```python
from build123d import *

# Parameters (mm, degrees)
BOSS_EXTRUDE1_DEPTH = 6.18
SKETCH2_R           = 2.1
CUT_EXTRUDE1_DEPTH  = 45.955560266
FILLET1_R           = 2
SKETCH3_R           = 1.16
BOSS_EXTRUDE2_DEPTH = 2
SKETCH5_W           = 46.23261583
SKETCH5_H           = 41.700006435
CUT_EXTRUDE2_DEPTH  = 6.18
SKETCH9_R           = 1.3
CUT_EXTRUDE3_DEPTH  = 39.857224753


with BuildPart() as part:
    # Sketch1 → Boss-Extrude1 (new body)
    with BuildSketch(Plane.XY):
        Polygon((0, 0), (0, 10), (7.5, 10), (12.499244943, 14.999244943), (12.499244943, 34.4), (24.749244943, 34.4), (24.749244943, 14.999244943), (29.748489886, 10), (37.248489886, 10), (37.248489886, 0), align=None)
    extrude(amount=BOSS_EXTRUDE1_DEPTH)

    # Sketch2 → Cut-Extrude1 (cut, through all)
    with BuildSketch(Plane(origin=(0, 10, 0), x_dir=(1, 0, 0), z_dir=(0, 1, 0))):
        with Locations(Location((3.75, -3.09, 0), (0, 0, 270))):
            Circle(SKETCH2_R)
        with Locations(Location((33.498489886, -3.09, 0), (0, 0, 270))):
            Circle(SKETCH2_R)
    extrude(amount=-CUT_EXTRUDE1_DEPTH, mode=Mode.SUBTRACT)

    # Fillet1
    fillet1_edges = [part.edges().sort_by_distance(p)[0] for p in [
        (0, 5, 0),
        (37.248489886, 5, 0),
        (12.499244943, 34.4, 3.09),
        (24.749244943, 34.4, 3.09),
        (0, 5, 6.18),
        (37.248489886, 5, 6.18),
    ]]
    fillet(fillet1_edges, radius=FILLET1_R)

    # Sketch3 → Boss-Extrude2 (add)
    # profile 1 of 15: a face of its own
    with BuildSketch(Plane(origin=(0, 0, 0), x_dir=(-1, 0, 0), z_dir=(0, 0, -1))):
        with BuildLine():
            Line((-14.76314253, 29.959470635), (-15.91314253, 29.959470635))
            ThreePointArc((-15.91314253, 29.959470635), (-18.51314253, 27.359470635), (-21.11314253, 29.959470635))
            Line((-21.11314253, 29.959470635), (-21.11314253, 21.454771123))
            Line((-21.11314253, 21.454771123), (-12.499244943, 21.454771123))
            Line((-12.499244943, 21.454771123), (-12.499244943, 22.849229594))
            ThreePointArc((-12.499244943, 22.849229594), (-13.32314253, 23.959470635), (-12.499244943, 25.069711675))
            Line((-12.499244943, 25.069711675), (-12.499244943, 27.381286163))
            ThreePointArc((-12.499244943, 27.381286163), (-14.116839829, 28.243933732), (-14.76314253, 29.959470635))
        make_face()
        with Locations((-18.51314253, 23.959470635)):
            Circle(SKETCH3_R, mode=Mode.SUBTRACT)
    # profile 2 of 15: a face of its own
    with BuildSketch(Plane(origin=(0, 0, 0), x_dir=(-1, 0, 0), z_dir=(0, 0, -1))):
        with BuildLine():
            ThreePointArc((-9.56314253, 29.959470635), (-10.447605628, 28.005773335), (-12.499244943, 27.381286163))
            Line((-12.499244943, 27.381286163), (-12.499244943, 25.069711675))
            ThreePointArc((-12.499244943, 25.069711675), (-11.47186791, 24.890995943), (-11.00314253, 23.959470635))
            ThreePointArc((-11.00314253, 23.959470635), (-11.47186791, 23.027945327), (-12.499244943, 22.849229594))
            Line((-12.499244943, 22.849229594), (-12.499244943, 21.454771123))
            Line((-12.499244943, 21.454771123), (-9.56314253, 21.454771123))
            Line((-9.56314253, 21.454771123), (-9.56314253, 29.959470635))
        make_face()
    # profile 3 of 15: a face of its own
    with BuildSketch(Plane(origin=(0, 0, 0), x_dir=(-1, 0, 0), z_dir=(0, 0, -1))):
        with BuildLine():
            Line((-13.31814253, 29.959470635), (-14.76314253, 29.959470635))
            ThreePointArc((-14.76314253, 29.959470635), (-14.116839829, 28.243933732), (-12.499244943, 27.381286163))
            Line((-12.499244943, 27.381286163), (-12.499244943, 28.854454722))
            ThreePointArc((-12.499244943, 28.854454722), (-13.091103544, 29.271783673), (-13.31814253, 29.959470635))
        make_face()
    # profile 4 of 15: a face of its own
    with BuildSketch(Plane(origin=(0, 0, 0), x_dir=(-1, 0, 0), z_dir=(0, 0, -1))):
        with BuildLine():
            Line((-12.499244943, 28.854454722), (-12.499244943, 27.381286163))
            ThreePointArc((-12.499244943, 27.381286163), (-10.447605628, 28.005773335), (-9.56314253, 29.959470635))
            Line((-9.56314253, 29.959470635), (-11.00814253, 29.959470635))
            ThreePointArc((-11.00814253, 29.959470635), (-11.475455569, 29.031509621), (-12.499244943, 28.854454722))
        make_face()
    # profile 5 of 15: a face of its own
    with BuildSketch(Plane(origin=(0, 0, 0), x_dir=(-1, 0, 0), z_dir=(0, 0, -1))):
        with BuildLine():
            Line((-13.31814253, 29.959470635), (-14.76314253, 29.959470635))
            ThreePointArc((-14.76314253, 29.959470635), (-14.116839829, 28.243933732), (-12.499244943, 27.381286163))
            Line((-12.499244943, 27.381286163), (-12.499244943, 28.854454722))
            ThreePointArc((-12.499244943, 28.854454722), (-13.091103544, 29.271783673), (-13.31814253, 29.959470635))
        make_face()
    # profile 6 of 15: a face of its own
    with BuildSketch(Plane(origin=(0, 0, 0), x_dir=(-1, 0, 0), z_dir=(0, 0, -1))):
        with BuildLine():
            Line((-12.499244943, 28.854454722), (-12.499244943, 27.381286163))
            ThreePointArc((-12.499244943, 27.381286163), (-10.447605628, 28.005773335), (-9.56314253, 29.959470635))
            Line((-9.56314253, 29.959470635), (-11.00814253, 29.959470635))
            ThreePointArc((-11.00814253, 29.959470635), (-11.475455569, 29.031509621), (-12.499244943, 28.854454722))
        make_face()
    # profile 7 of 15: a face of its own
    with BuildSketch(Plane(origin=(0, 0, 0), x_dir=(-1, 0, 0), z_dir=(0, 0, -1))):
        with BuildLine():
            ThreePointArc((-13.104419545, 32.383103771), (-14.308756689, 31.427918755), (-14.76314253, 29.959470635))
            Line((-14.76314253, 29.959470635), (-13.31814253, 29.959470635))
            ThreePointArc((-13.31814253, 29.959470635), (-13.091103544, 30.647157596), (-12.499244943, 31.064486548))
            Line((-12.499244943, 31.064486548), (-12.499244943, 32.4))
            ThreePointArc((-12.499244943, 32.4), (-12.500420382, 32.468559287), (-12.503945319, 32.537037988))
            ThreePointArc((-12.503945319, 32.537037988), (-12.808786466, 32.478030522), (-13.104419545, 32.383103771))
        make_face()
    # profile 8 of 15: a face of its own
    with BuildSketch(Plane(origin=(0, 0, 0), x_dir=(-1, 0, 0), z_dir=(0, 0, -1))):
        with BuildLine():
            Line((-12.499244943, 32.4), (-12.499244943, 31.064486548))
            ThreePointArc((-12.499244943, 31.064486548), (-11.475455569, 30.887431649), (-11.00814253, 29.959470635))
            Line((-11.00814253, 29.959470635), (-9.56314253, 29.959470635))
            ThreePointArc((-9.56314253, 29.959470635), (-10.449387479, 31.914731135), (-12.503945319, 32.537037988))
            ThreePointArc((-12.503945319, 32.537037988), (-12.500420382, 32.468559287), (-12.499244943, 32.4))
        make_face()
    # profile 9 of 15: a face of its own
    with BuildSketch(Plane(origin=(0, 0, 0), x_dir=(-1, 0, 0), z_dir=(0, 0, -1))):
        with BuildLine():
            ThreePointArc((-13.104419545, 32.383103771), (-14.308756689, 31.427918755), (-14.76314253, 29.959470635))
            Line((-14.76314253, 29.959470635), (-13.31814253, 29.959470635))
            ThreePointArc((-13.31814253, 29.959470635), (-13.091103544, 30.647157596), (-12.499244943, 31.064486548))
            Line((-12.499244943, 31.064486548), (-12.499244943, 32.4))
            ThreePointArc((-12.499244943, 32.4), (-12.500420382, 32.468559287), (-12.503945319, 32.537037988))
            ThreePointArc((-12.503945319, 32.537037988), (-12.808786466, 32.478030522), (-13.104419545, 32.383103771))
        make_face()
    # profile 10 of 15: a face of its own
    with BuildSketch(Plane(origin=(0, 0, 0), x_dir=(-1, 0, 0), z_dir=(0, 0, -1))):
        with BuildLine():
            Line((-12.499244943, 32.4), (-12.499244943, 31.064486548))
            ThreePointArc((-12.499244943, 31.064486548), (-11.475455569, 30.887431649), (-11.00814253, 29.959470635))
            Line((-11.00814253, 29.959470635), (-9.56314253, 29.959470635))
            ThreePointArc((-9.56314253, 29.959470635), (-10.449387479, 31.914731135), (-12.503945319, 32.537037988))
            ThreePointArc((-12.503945319, 32.537037988), (-12.500420382, 32.468559287), (-12.499244943, 32.4))
        make_face()
    # profile 11 of 15: a face of its own
    with BuildSketch(Plane(origin=(0, 0, 0), x_dir=(-1, 0, 0), z_dir=(0, 0, -1))):
        with BuildLine():
            ThreePointArc((-19.66814253, 29.959470635), (-18.51314253, 31.114470635), (-17.35814253, 29.959470635))
            Line((-17.35814253, 29.959470635), (-15.91314253, 29.959470635))
            ThreePointArc((-15.91314253, 29.959470635), (-16.367528354, 31.42791873), (-17.571865459, 32.38310375))
            ThreePointArc((-17.571865459, 32.38310375), (-19.981590625, 32.105084811), (-21.11314253, 29.959470635))
            Line((-21.11314253, 29.959470635), (-19.66814253, 29.959470635))
        make_face()
    # profile 12 of 15: a face of its own
    with BuildSketch(Plane(origin=(0, 0, 0), x_dir=(-1, 0, 0), z_dir=(0, 0, -1))):
        with BuildLine():
            Line((-15.91314253, 29.959470635), (-17.35814253, 29.959470635))
            ThreePointArc((-17.35814253, 29.959470635), (-18.51314253, 28.804470635), (-19.66814253, 29.959470635))
            Line((-19.66814253, 29.959470635), (-21.11314253, 29.959470635))
            ThreePointArc((-21.11314253, 29.959470635), (-18.51314253, 27.359470635), (-15.91314253, 29.959470635))
        make_face()
    # profile 13 of 15: a face of its own
    with BuildSketch(Plane(origin=(0, 0, 0), x_dir=(-1, 0, 0), z_dir=(0, 0, -1))):
        with BuildLine():
            ThreePointArc((-19.66814253, 29.959470635), (-18.51314253, 31.114470635), (-17.35814253, 29.959470635))
            Line((-17.35814253, 29.959470635), (-15.91314253, 29.959470635))
            ThreePointArc((-15.91314253, 29.959470635), (-16.367528354, 31.42791873), (-17.571865459, 32.38310375))
            ThreePointArc((-17.571865459, 32.38310375), (-19.981590625, 32.105084811), (-21.11314253, 29.959470635))
            Line((-21.11314253, 29.959470635), (-19.66814253, 29.959470635))
        make_face()
    # profile 14 of 15: a face of its own
    with BuildSketch(Plane(origin=(0, 0, 0), x_dir=(-1, 0, 0), z_dir=(0, 0, -1))):
        with BuildLine():
            Line((-15.91314253, 29.959470635), (-17.35814253, 29.959470635))
            ThreePointArc((-17.35814253, 29.959470635), (-18.51314253, 28.804470635), (-19.66814253, 29.959470635))
            Line((-19.66814253, 29.959470635), (-21.11314253, 29.959470635))
            ThreePointArc((-21.11314253, 29.959470635), (-18.51314253, 27.359470635), (-15.91314253, 29.959470635))
        make_face()
    # profile 15 of 15: a face of its own
    with BuildSketch(Plane(origin=(0, 0, 0), x_dir=(-1, 0, 0), z_dir=(0, 0, -1))):
        with BuildLine():
            ThreePointArc((-17.571865459, 32.38310375), (-16.367528354, 31.42791873), (-15.91314253, 29.959470635))
            Line((-15.91314253, 29.959470635), (-14.76314253, 29.959470635))
            ThreePointArc((-14.76314253, 29.959470635), (-14.308756689, 31.427918755), (-13.104419545, 32.383103771))
            ThreePointArc((-13.104419545, 32.383103771), (-15.3381425, 31.964571551), (-17.571865459, 32.38310375))
        make_face()
    extrude(amount=BOSS_EXTRUDE2_DEPTH)

    # Sketch5 → Cut-Extrude2 (cut)
    with BuildSketch(Plane.XY.offset(6.18)):
        with Locations((18.136117777, 17.095401322)):
            Rectangle(SKETCH5_W, SKETCH5_H)
    extrude(amount=-CUT_EXTRUDE2_DEPTH, mode=Mode.SUBTRACT)

    # Sketch9 → Cut-Extrude3 (cut, through all)
    with BuildSketch(Plane(origin=(0, 0, -2), x_dir=(-1, 0, 0), z_dir=(0, 0, -1))):
        with Locations((-18.51314253, 29.959470635)):
            Circle(SKETCH9_R)
        with Locations((-12.16314253, 29.959470635)):
            Circle(SKETCH9_R)
    extrude(amount=-CUT_EXTRUDE3_DEPTH, mode=Mode.SUBTRACT)


solid = part.part
```
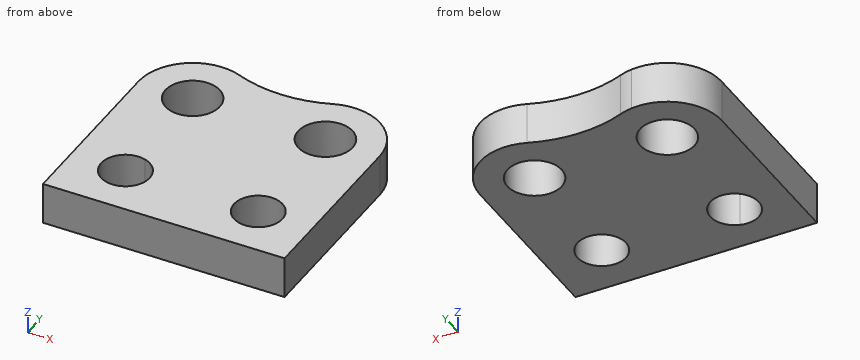
Source: CAD feature listing. Evaluate the final solid. Frame: model axes, mm. Round coordinates to 2 decimals unless told otherwise and drop trailing zeros. Write each loop counter-clockwise with the first axis right and the second up, starting at its lowest first coordinate (ties: lowest second). Pieces come first, ordered by that corner, then holes. Notation, with made-up numbers: M 44.5,66.25 L 51.5,66.25 A20 cw 51.5,87.25 Z; hole C -19,75 d3. An arc over 180 degrees is marked long. Use CSV: the item, a comma, the result in double quotes. Start each with the question number.
Q1. First-contact query: P1, Ø1, axis at x = 17.5, z = -0.5, coming from the +Y side; P2, Ø2, axis at x = 18.51, y = 29.96, coming from the -Z side; P3, Ø1, axis at x = 20, z = -1, coming from the +Y side. Flat tips, straight axial feed; report the tip coordinate or a pass-through.
Q2. Cut plane D-D on x = 14.25. Output: boundary loops of the cut face in (y, z).
Q3. Line query: line 1 (X direction, y = 29.25, z = -1.85); line 2 (X direction, y = 23.5, z = -1.15); line 3 (Y direction, x = 17.75, z = -1.35). Output: solid intervals per line, ascending. Write a range as from..to.
Q4. Cut plane A-A on z = -1.05. Output: boundary loops of the cut face in (x, y).
Q5. Cut plane B-B on y = 29.5. Output: boundary loops of the cut face in (x, z), plus the area to 3 significant figures.
Q6. Cut plane C-C on x = 11.25. Output: boundary loops of the cut face in (y, z).
Results found:
1,P1,"y = 32.51"
1,P2,"through"
1,P3,"y = 32.36"
2,outline,"M 21.45,-2 L 32.06,-2 L 32.06,0 L 21.45,0 Z"
3,line 1,"9.56..11.07, 13.25..17.42, 19.6..21.11"
3,line 2,"9.56..11.1, 13.23..17.45, 19.58..21.11"
3,line 3,"21.45..23.09, 24.83..28.91, 31.01..32.44"
4,outline,"M 9.56,21.45 L 21.11,21.45 L 21.11,29.96 A2.6 ccw 17.57,32.38 A6.17 cw 13.1,32.38 A2.6 ccw 9.56,29.96 Z; hole C 12.16,29.96 d2.6; hole C 12.16,23.96 d2.32; hole C 18.51,29.96 d2.6; hole C 18.51,23.96 d2.32"
5,outline,"M 9.56,-2 L 10.95,-2 L 10.95,0 L 9.56,0 Z; M 13.38,-2 L 17.3,-2 L 17.3,0 L 13.38,0 Z; M 19.73,-2 L 21.11,-2 L 21.11,0 L 19.73,0 Z"
5,area,"13.4 mm^2"
6,outline,"M 21.45,-2 L 23.24,-2 L 23.24,0 L 21.45,0 Z; M 24.67,-2 L 29.03,-2 L 29.03,0 L 24.67,0 Z; M 30.88,-2 L 32.39,-2 L 32.39,0 L 30.88,0 Z"
